Here's how the part is built. I have some questions about the finished solid (model axes, mm). A direction names the side the tool comes from. Give positions to 0.01 mm unless a question says otherwise; leave off trailing zeros. Write each loop counter-clockwise with the first axis right and the second up, starting at its lowest first coordinate (ties: lowest second). Pieces come first, ordered by that corner, then holes. Notation, with made-up numbers: (-37.75, 56) -> (6.25, 56) arc R30 cw to (6.25, 93) -> close; hole circle Ø10 at (-17, -18.5). An arc over 180 degrees is marked (long way). Use one line per item in the form item = value.
```python
from build123d import *

# Parameters (mm, degrees)
CYLINDER097_R     = 3.5
CYLINDER097_DEPTH = 4
CYLINDER098_R     = 1.5
CYLINDER098_DEPTH = 25
CYLINDER096_R     = 3.5
CYLINDER096_DEPTH = 4
CYLINDER095_R     = 1.5
CYLINDER095_DEPTH = 25
CYLINDER093_R     = 3.5
CYLINDER093_DEPTH = 20
BOX030_W          = 20
BOX030_H          = 11
BOX030_DEPTH      = 10.3
BOX029_W          = 20
BOX029_H          = 11
BOX029_DEPTH      = 10.3
BOX027_W          = 20
BOX027_H          = 14
BOX027_DEPTH      = 12.2
BOX028_W          = 20
BOX028_H          = 14
BOX028_DEPTH      = 12.2
BOX026_W          = 20
BOX026_H          = 46
BOX026_DEPTH      = 10
CYLINDER094_R     = 9.5
CYLINDER094_DEPTH = 20


with BuildPart() as zylinder094:
    # Cylinder097 → Cylinder097 (new body)
    with BuildSketch(Plane.XY):
        Circle(CYLINDER097_R)
    extrude(amount=CYLINDER097_DEPTH)


with BuildPart() as fusion034:
    # Cylinder098 → Cylinder098 (new body)
    with BuildSketch(Plane.XY):
        Circle(CYLINDER098_R)
    extrude(amount=CYLINDER098_DEPTH)

    # Fusion034: union Zylinder094
    add(zylinder094.part)


with BuildPart() as fusion034_1:
    # Fusion034 placement: moved
    add(fusion034.part.moved(Location((-13, 16, 58))))


with BuildPart() as zylinder093:
    # Cylinder096 → Cylinder096 (new body)
    with BuildSketch(Plane.XY):
        Circle(CYLINDER096_R)
    extrude(amount=CYLINDER096_DEPTH)


with BuildPart() as fusion035:
    # Cylinder095 → Cylinder095 (new body)
    with BuildSketch(Plane.XY):
        Circle(CYLINDER095_R)
    extrude(amount=CYLINDER095_DEPTH)

    # Fusion033: union Zylinder093
    add(zylinder093.part)


with BuildPart() as fusion035_1:
    # Fusion033 placement: moved
    add(fusion035.part.moved(Location((-13, -16, 58))))

    # Fusion035: union Fusion034
    add(fusion034_1.part)


with BuildPart() as zylinder090:
    # Cylinder093 → Cylinder093 (new body)
    with BuildSketch(Plane(origin=(-23, 0, 63), x_dir=(0, 0, -1), z_dir=(1, 0, 0))):
        Circle(CYLINDER093_R)
    extrude(amount=CYLINDER093_DEPTH)


with BuildPart() as obj1:
    # Box030 → Box030 (new body)
    with BuildSketch(Plane(origin=(-23, -21.5, 68), x_dir=(1, 0, 0), z_dir=(0, 0, 1))):
        with Locations((10, 5.5)):
            Rectangle(BOX030_W, BOX030_H)
    extrude(amount=BOX030_DEPTH)


with BuildPart() as fusion030:
    # Box029 → Box029 (new body)
    with BuildSketch(Plane(origin=(-23, 10.5, 68), x_dir=(1, 0, 0), z_dir=(0, 0, 1))):
        with Locations((10, 5.5)):
            Rectangle(BOX029_W, BOX029_H)
    extrude(amount=BOX029_DEPTH)

    # Fusion030: union obj1
    add(obj1.part)


with BuildPart() as obj2:
    # Box027 → Box027 (new body)
    with BuildSketch(Plane(origin=(-23, 9, 68), x_dir=(1, 0, 0), z_dir=(0, 0, 1))):
        with Locations((10, 7)):
            Rectangle(BOX027_W, BOX027_H)
    extrude(amount=BOX027_DEPTH)


with BuildPart() as cut047:
    # Box028 → Box028 (new body)
    with BuildSketch(Plane(origin=(-23, -23, 68), x_dir=(1, 0, 0), z_dir=(0, 0, 1))):
        with Locations((10, 7)):
            Rectangle(BOX028_W, BOX028_H)
    extrude(amount=BOX028_DEPTH)

    # Fusion029: union obj2
    add(obj2.part)

    # Cut047: cut Fusion030
    add(fusion030.part, mode=Mode.SUBTRACT)


with BuildPart() as fusion031:
    # Box026 → Box026 (new body)
    with BuildSketch(Plane(origin=(-23, -23, 58), x_dir=(1, 0, 0), z_dir=(0, 0, 1))):
        with Locations((10, 23)):
            Rectangle(BOX026_W, BOX026_H)
    extrude(amount=BOX026_DEPTH)

    # Fusion031: union Cut047
    add(cut047.part)


with BuildPart() as belt_tensioner:
    # Cylinder094 → Cylinder094 (new body)
    with BuildSketch(Plane(origin=(-23, 0, 63), x_dir=(0, 0, -1), z_dir=(1, 0, 0))):
        Circle(CYLINDER094_R)
    extrude(amount=CYLINDER094_DEPTH)

    # Fusion032: union Fusion031
    add(fusion031.part)

    # Cut048: cut Zylinder090
    add(zylinder090.part, mode=Mode.SUBTRACT)

    # Cut049: cut Fusion035
    add(fusion035_1.part, mode=Mode.SUBTRACT)


solid = belt_tensioner.part
```
Q1. If we mould it in two halves opening along Z, with no side actions, what happens to faces 1 (the face through (-13, 10.5, 73)), 2 (the face through (-13, 14, 62)), 3 (the face through (-13, -9, 74))? For each: +Z half, -Z half, draft (parallel to the pull), parting line (faces both ways), or undercut.
Result set:
face_1 = undercut
face_2 = -Z half
face_3 = draft
Q2. I want a section at B-B, the plane y = 0. Write out the boundary of the cut face in (x, z), and give its area (3 significant figures).
Result set:
outline = (-23, 53.5) -> (-3, 53.5) -> (-3, 59.5) -> (-23, 59.5) -> close; (-23, 66.5) -> (-3, 66.5) -> (-3, 72.5) -> (-23, 72.5) -> close
area = 240 mm2
Q3. I want a section at C-C, the plane z = 76.5. Write out the boundary of the cut face in (x, y), and give its area (3 significant figures).
Result set:
outline = (-23, -23) -> (-3, -23) -> (-3, -21.5) -> (-23, -21.5) -> close; (-23, -10.5) -> (-3, -10.5) -> (-3, -9) -> (-23, -9) -> close; (-23, 9) -> (-3, 9) -> (-3, 10.5) -> (-23, 10.5) -> close; (-23, 21.5) -> (-3, 21.5) -> (-3, 23) -> (-23, 23) -> close
area = 120 mm2
Q4. If I drill on line 1 along Y through (x, z) = (-11.5, 74.75); line 2 along Y through (x, z) = (-13, 79.3); line 3 along X through (y, z) = (-16, 79.55), over which ranges is the centre line in solid material (lowest first)? Write a range as from..to.
Result set:
line_1 = -23..-21.5, -10.5..-9, 9..10.5, 21.5..23
line_2 = -23..-17.5, -14.5..-9, 9..14.5, 17.5..23
line_3 = -23..-14.5, -11.5..-3
Q5. I want a section at D-D, the plane x = -20.5. Write out the boundary of the cut face in (y, z), and give its area (3 significant figures).
Result set:
outline = (-23, 58) -> (-8.08, 58) arc R9.5 ccw to (8.08, 58) -> (23, 58) -> (23, 80.2) -> (9, 80.2) -> (9, 68) -> (8.08, 68) arc R9.5 ccw to (-8.08, 68) -> (-9, 68) -> (-9, 80.2) -> (-23, 80.2) -> close; hole (-21.5, 68) -> (-10.5, 68) -> (-10.5, 78.3) -> (-21.5, 78.3) -> close; hole circle Ø7 at (0, 63); hole (10.5, 68) -> (21.5, 68) -> (21.5, 78.3) -> (10.5, 78.3) -> close
area = 639 mm2
Q6. I want a section at A-A, the plane z = 63. Write out the boundary of the cut face in (x, y), and give its area (3 significant figures).
Result set:
outline = (-23, -23) -> (-3, -23) -> (-3, -3.5) -> (-23, -3.5) -> close; (-23, 3.5) -> (-3, 3.5) -> (-3, 23) -> (-23, 23) -> close; hole circle Ø3 at (-13, -16); hole circle Ø3 at (-13, 16)
area = 766 mm2
Q7. Will these pins go through, and if not, where does the flat tip stop? pin 1 Ø0.5 at (x, y) = (-8.5, 8.5) entering from +Z; pin 2 Ø9 at (x, y) = (-16, 14.5) entering from -Z; pin 3 Ø3.5 at (x, y) = (-13, 16) entering from -Z.
Result set:
pin_1 = 68
pin_2 = 58
pin_3 = 62
Q8. Which directions (+Z, -Z, +X, -X, +Y, -Y) give clear straight access to the entire face, cutting with the end or side of a thin tool? Please do faces 4 (the face through (-13, 9, 74)), 5 (the face through (-15, 16, 78.3)), 6 (the face through (-13, 12, 58)), 7 (the face through (-11.385, -19.105, 59.972)).
Result set:
face_4 = +Z, +X, -X
face_5 = +X, -X
face_6 = -Z, +X, -X, +Y
face_7 = -Z
